Here's how the part is built. I have some questions about the finished solid (model axes, mm). A direction names the side the tool comes from. Give positions to 0.01 mm unless a question says otherwise; leave off trailing zeros. Loops run counter-clockwise (first coordinate to the right, second up) from the corner with the lowest first, then second, coordinate; pieces in that order, holes last. Notation, with made-up numbers: (-12, 82) - (27, 82) arc R17 ccw to (27, 87) - close; hole circle Ø10 at (-20.75, -4). An arc over 180 degrees is marked (long way). One line per item, written item: value. Start each with the question number.
```python
from build123d import *

# Parameters (mm, degrees)
F0_W     = 114.3
F0_H     = 114.3
F1_DEPTH = 228.6
F2_T     = -0.8
F3_R     = 1
F4_DEPTH = 25.4
F5_W     = 8
F5_H     = 2
F6_DEPTH = 114.301
F7_W     = 8
F7_H     = 4
F8_DEPTH = 114.301


with BuildPart() as f1:
    # F0 (on Top) → F1 (new body)
    with BuildSketch(Plane.XY):
        Rectangle(F0_W, F0_H)
    extrude(amount=F1_DEPTH)

    # F2
    f2_openings = [f1.faces().sort_by_distance(p)[0] for p in [
        (0, 0, 228.6),
    ]]
    offset(amount=F2_T, openings=f2_openings)

    # F3 (on face) → F4 (cut)
    with BuildSketch(Plane.XY.offset(0.8)):
        Circle(F3_R)
    extrude(amount=-F4_DEPTH, mode=Mode.SUBTRACT)

    # F5 (on face) → F6 (cut, through all)
    with BuildSketch(Plane.XZ.offset(57.15)):
        with Locations((0, 227.6)):
            Rectangle(F5_W, F5_H)
    extrude(amount=-F6_DEPTH, mode=Mode.SUBTRACT)

    # F7 (on face) → F8 (cut, through all)
    with BuildSketch(Plane.YZ.offset(57.15)):
        with Locations((0, 226.6)):
            Rectangle(F7_W, F7_H)
    extrude(amount=-F8_DEPTH, mode=Mode.SUBTRACT)


solid = f1.part
```
(1) Please list where these lines run through material, in increasing order: probe 1 along X at (y, z) = (11, 216.5); probe 2 along Y at (x, z) = (0, 0.65). Write a range as from..to.
(2) If we mould it in two halves opening along Y, with no side actions, what happens to faces 1 (the face through (-1, 56.35, 113)), 2 (the face through (-1, 1, 0)), 3 (the face through (-56.35, -1, 113)), 4 (the face through (-1, -57.15, 113))? For each: pulls with the +Y half, pulls with the -Y half, needs draft (parallel to the pull), parting line crosses it, or undercut.
(3) Will these pins go through, and if not, where does the flat tip stop? pin 1 (8 mm diameter, centred on x = -6.5, y = -13, fed in from +Z); pin 2 (1.2 mm diameter, centred on x = 0, y = 0, fed in from -Z); pin 3 (1.5 mm diameter, centred on x = 5.5, y = -18.5, fed in from -Z); pin 4 (0.6 mm diameter, centred on x = -57, y = 0, fed in from +Z).
(4) If we section it at B-B on x = -7: List the corners of the cut face in (y, z) for me.
(5) If we section it at A-A on z = 73.5: List the corners of the cut face in (x, y) for me, plus the area to 3 significant figures.
(6) For faces 5 (the face through (57.15, -1, 113)), 6 (the face through (-1, 1, 0.8)), which set-ups out of +Z, -Z, +X, -X, +Y, -Y let a thin tool reach every point of the face, with its end or its side?
Found:
1. probe 1: -57.15..-56.35, 56.35..57.15
1. probe 2: -57.15..-1, 1..57.15
2. face 1: undercut
2. face 2: needs draft
2. face 3: undercut
2. face 4: pulls with the -Y half
3. pin 1: z = 0.8
3. pin 2: through
3. pin 3: z = 0
3. pin 4: z = 224.6
4. outline: (-57.15, 0) - (57.15, 0) - (57.15, 228.6) - (56.35, 228.6) - (56.35, 0.8) - (-56.35, 0.8) - (-56.35, 228.6) - (-57.15, 228.6) - close
5. outline: (-57.15, -57.15) - (57.15, -57.15) - (57.15, 57.15) - (-57.15, 57.15) - close; hole (-56.35, -56.35) - (56.35, -56.35) - (56.35, 56.35) - (-56.35, 56.35) - close
5. area: 363 mm^2
6. face 5: +Z, -Z, +X, +Y, -Y
6. face 6: +Z
